Could you check a few things on this model? Use its own coordinates, in mm. A direction names the side the tool comes from. Give positions to 0.01 mm unless a question says otherwise; leave off trailing zeros. Order: outer loops, then holes, each group sorted by start corner. A loop starts at its lowest first (then second) coordinate and runs counter-clockwise, first axis right, second up. Notation, with made-up numbers: (-35, -12) - (4, -12) arc R16 ccw to (4, 12) - close; hole circle Ø3 at (51, -7.75). An arc over 180 degrees is marked (long way). One line per question, with ' | ' between items. Start each with the question number.
1. Which directions (+Z, -Z, +X, -X, +Y, -Y) give clear straight access to the entire face, cutting with the end or side of a thin tool? Please do faces 5 (the flat face through (-4.5, -2.6, 13.1)), 6 (the flat face through (-3.216, -1.822, 14.26)), 7 (the flat face through (1, 4, -12)), 8 (the cylindrical face through (-4.28, -2.52, -14.79)), 9 (the flat face through (3.19, -1.87, -14.26)).
2. For P1, Ø3, axis at x = -0.5, y = -1.5, coming from the +Z side; P2, Ø1.5, axis at y = 2, z = -1.5, coming from the -X side; P3, Ø2, axis at x = 2, y = 3.5, coming from the -Z side; P4, Ø1, axis at x = 1, z = -6.5, coming from the +Y side, each with a flat end and sliding along its axis, tell me the tip position at first contact or that it passes through.
3. Imagine slicing it at B-B (z = -10). Please give me the cut outline in (x, y), and give its area (3 significant figures).
4. I need wall thicknesses on probe 1 along Z at (x, y) = (4.5, -1.25); probe 2 along X at (y, z) = (2.25, -4); probe 3 along Z at (x, y) = (-0.5, 1). Which ranges of each line are inside material? Lowest first, please. Write a range as from..to.
5. If we mould it in two halves opening along Y, with no side actions, what happens to faces 1 (the flat face through (0, -5.196, 13)), 2 (the flat face through (0, 3.696, -14)), 3 (the flat face through (1, 4, 12)), 4 (the cylindrical face through (4.294, 2.528, 14.774))? For each: released by +Y, released by -Y, zero draft, split by the parting line, or undercut.
6. Imagine slicing it at A-A (x = 0). Please give me the cut outline in (y, z), and give its area (3 significant figures).
```python
from build123d import *

# Parameters (mm, degrees)
BOSS_EXTRUDE1_DEPTH      = 2
BOSS_EXTRUDE1_DEPTH_BACK = 2
SKETCH1_R                = 0.625
BOSS_EXTRUDE2_DEPTH      = 0.5
FILLET1_R                = 0.125
CUT_EXTRUDE2_DEPTH       = 0.25
FILLET1_OF_MIRROR1_R     = 0.125
SCALE1_SCALE             = 6


with BuildPart() as part:
    # Sketch1 → Boss-Extrude1 (new, two sides: drawn at the far end of the back side and taken through both)
    with BuildSketch(Plane.XY.offset(-BOSS_EXTRUDE1_DEPTH_BACK)):
        Circle(SKETCH1_R)
    extrude(amount=BOSS_EXTRUDE1_DEPTH + BOSS_EXTRUDE1_DEPTH_BACK)

    # Sketch2 → Boss-Extrude2 (add)
    with BuildSketch(Plane.XY.offset(2)):
        Polygon((1, 0), (0.5, 0.866025404), (-0.5, 0.866025404), (-1, 0), (-0.5, -0.866025404), (0.5, -0.866025404), align=None)
    boss_extrude2 = extrude(amount=BOSS_EXTRUDE2_DEPTH)

    # Fillet1
    fillet1_edges = [part.edges().sort_by_distance(p)[0] for p in [
        (0.75, -0.433012702, 2.5),
        (0.75, 0.433012702, 2.5),
        (0, 0.866025404, 2.5),
        (-0.75, 0.433012702, 2.5),
        (-0.75, -0.433012702, 2.5),
        (0, -0.866025404, 2.5),
    ]]
    fillet(fillet1_edges, radius=FILLET1_R)

    # Sketch6 → Cut-Extrude2 (cut)
    with BuildSketch(Plane.XY.offset(2.5)):
        Polygon((-0.711324865, 0), (-0.355662433, -0.616025404), (0.355662433, -0.616025404), (0.711324865, 0), (0.355662433, 0.616025404), (-0.355662433, 0.616025404), align=None)
    cut_extrude2 = extrude(amount=-CUT_EXTRUDE2_DEPTH, mode=Mode.SUBTRACT)

    # Mirror1: Boss-Extrude2, Cut-Extrude2 across plane
    add(boss_extrude2.mirror(Plane.XY))
    add(cut_extrude2.mirror(Plane.XY), mode=Mode.SUBTRACT)

    # Fillet1 of Mirror1
    fillet1_of_mirror1_edges = [part.edges().sort_by_distance(p)[0] for p in [
        (0.75, -0.433012702, -2.5),
        (0.75, 0.433012702, -2.5),
        (0, 0.866025404, -2.5),
        (-0.75, 0.433012702, -2.5),
        (-0.75, -0.433012702, -2.5),
        (0, -0.866025404, -2.5),
    ]]
    fillet(fillet1_of_mirror1_edges, radius=FILLET1_OF_MIRROR1_R)


with BuildPart() as part_1:
    # Scale1: scaled about (0, 0, 0)
    add(part.part.scale(SCALE1_SCALE))


solid = part_1.part
```
Results found:
1) face 5: +Z, -Z, -X, -Y | face 6: +Z | face 7: none | face 8: -Z, -X, -Y | face 9: -Z
2) P1: stops at z = 13.5 | P2: stops at x = -3.54 | P3: stops at z = -15 | P4: stops at y = 3.72
3) outline: circle Ø7.5 at (0, 0) | area: 44.2 mm2
4) probe 1: z = -15..-12, 12..15 | probe 2: x = -3..3 | probe 3: z = -13.5..13.5
5) face 1: released by -Y | face 2: undercut | face 3: zero draft | face 4: released by +Y
6) outline: (-5.2, -14.25) arc R0.75 ccw to (-4.45, -15) - (-3.7, -15) - (-3.7, -13.5) - (3.7, -13.5) - (3.7, -15) - (4.45, -15) arc R0.75 ccw to (5.2, -14.25) - (5.2, -12) - (3.75, -12) - (3.75, 12) - (5.2, 12) - (5.2, 14.25) arc R0.75 ccw to (4.45, 15) - (3.7, 15) - (3.7, 13.5) - (-3.7, 13.5) - (-3.7, 15) - (-4.45, 15) arc R0.75 ccw to (-5.2, 14.25) - (-5.2, 12) - (-3.75, 12) - (-3.75, -12) - (-5.2, -12) - close | area: 220 mm2
